Input: part model. Units: mm. Frame: model coordinates. A direction names the side the tool comes from. Round coordinates to 2 decimals unless told otherwise and drop trailing zeros. Order: outer loops, then holes, each group sorted by start corner. A loop starts at its lowest first (then second) coordinate and runs counter-clockwise, first axis right, second up. Notation, with made-up numbers: (59.25, 27) -> (68.25, 27) arc R23 ccw to (68.25, 47) -> close; hole circle Ø9 at (31, 87). An arc over 180 degrees is marked (long way). Use a Markdown table: item, result.
from build123d import *

# Parameters (mm, degrees)
SKETCH1_W           = 42
SKETCH1_H           = 47
BOSS_EXTRUDE1_DEPTH = 5
SKETCH4_W           = 42
SKETCH4_H           = 45
BOSS_EXTRUDE2_DEPTH = 5
BOSS_EXTRUDE3_DEPTH = 3
BOSS_EXTRUDE4_DEPTH = 3
SKETCH2_R           = 2.5
SKETCH2_R_2         = 4.5
CUT_EXTRUDE1_DEPTH  = 54.415821626
SKETCH9_R           = 2
CUT_EXTRUDE4_DEPTH  = 69.373971656
CHAMFER2_SIZE       = 3
CUT_EXTRUDE5_REACH  = 73.903
SKETCH10_R          = 1.5


with BuildPart() as part:
    # Sketch1 → Boss-Extrude1 (new body)
    with BuildSketch(Plane(origin=(0, 0, 0), x_dir=(1, 0, 0), z_dir=(0, 1, 0))):
        Rectangle(SKETCH1_W, SKETCH1_H)
    extrude(amount=BOSS_EXTRUDE1_DEPTH)

    # Sketch4 → Boss-Extrude2 (add)
    with BuildSketch(Plane(origin=(0, 0, -23.5), x_dir=(-1, 0, 0), z_dir=(0, 0, -1))):
        with Locations((0, 22.5)):
            Rectangle(SKETCH4_W, SKETCH4_H)
    extrude(amount=BOSS_EXTRUDE2_DEPTH)

    # Sketch5 → Boss-Extrude3 (add)
    with BuildSketch(Plane(origin=(21, 0, 0), x_dir=(0, 0, -1), z_dir=(1, 0, 0))):
        Polygon((23.5, 13), (15.5, 5), (23.5, 5), align=None)
    extrude(amount=-BOSS_EXTRUDE3_DEPTH)

    # Sketch6 → Boss-Extrude4 (add)
    with BuildSketch(Plane.ZY.offset(21)):
        Polygon((-23.5, 13), (-15.5, 5), (-23.5, 5), align=None)
    extrude(amount=-BOSS_EXTRUDE4_DEPTH)

    # Sketch2 → Cut-Extrude1 (cut, through all)
    with BuildSketch(Plane(origin=(0, 5, 0), x_dir=(1, 0, 0), z_dir=(0, 1, 0))):
        with Locations(Location((-13.081475452, 10.581475452, 0), (0, 0, 270))):
            Circle(SKETCH2_R)
        with Locations(Location((13.081475452, -15.581475452, 0), (0, 0, 270))):
            Circle(SKETCH2_R)
        with Locations(Location((0, -2.5, 0), (0, 0, 270))):
            Circle(SKETCH2_R_2)
    extrude(amount=-CUT_EXTRUDE1_DEPTH, mode=Mode.SUBTRACT)

    # Sketch9 → Cut-Extrude4 (cut, through all)
    with BuildSketch(Plane.XY.offset(-23.5)):
        with Locations((-12.5, 37.5)):
            Circle(SKETCH9_R)
        with Locations((12.5, 37.5)):
            Circle(SKETCH9_R)
        with Locations((12.5, 12.5)):
            Circle(SKETCH9_R)
        with Locations((-12.5, 12.5)):
            Circle(SKETCH9_R)
    extrude(amount=-CUT_EXTRUDE4_DEPTH, mode=Mode.SUBTRACT)

    # Chamfer2
    chamfer2_edges = [part.edges().sort_by_distance(p)[0] for p in [
        (-21, 2.5, 23.5),
        (21, 2.5, 23.5),
        (21, 45, -26),
        (-21, 45, -26),
    ]]
    chamfer(chamfer2_edges, length=CHAMFER2_SIZE)

    # Sketch10 → Cut-Extrude5 (cut, up to next)
    with BuildSketch(Plane(origin=(0, 0, -28.5), x_dir=(-1, 0, 0), z_dir=(0, 0, -1)), mode=Mode.PRIVATE) as cut_extrude5_sk1:
        with Locations((0, 25)):
            Circle(SKETCH10_R)
    cut_extrude5_tool1 = extrude(cut_extrude5_sk1.sketch, amount=-CUT_EXTRUDE5_REACH, mode=Mode.PRIVATE) & part.part
    # Sketch10 → Cut-Extrude5 (cut, up to next)
    with BuildSketch(Plane(origin=(0, 0, -28.5), x_dir=(-1, 0, 0), z_dir=(0, 0, -1)), mode=Mode.PRIVATE) as cut_extrude5_sk2:
        with Locations((0, 10)):
            Circle(SKETCH10_R)
    cut_extrude5_tool2 = extrude(cut_extrude5_sk2.sketch, amount=-CUT_EXTRUDE5_REACH, mode=Mode.PRIVATE) & part.part
    # Sketch10 → Cut-Extrude5 (cut, up to next)
    with BuildSketch(Plane(origin=(0, 0, -28.5), x_dir=(-1, 0, 0), z_dir=(0, 0, -1)), mode=Mode.PRIVATE) as cut_extrude5_sk3:
        with Locations((0, 40)):
            Circle(SKETCH10_R)
    cut_extrude5_tool3 = extrude(cut_extrude5_sk3.sketch, amount=-CUT_EXTRUDE5_REACH, mode=Mode.PRIVATE) & part.part
    add(cut_extrude5_tool1.solids().sort_by_distance((0, 25, -28.5))[0], mode=Mode.SUBTRACT)
    add(cut_extrude5_tool2.solids().sort_by_distance((0, 10, -28.5))[0], mode=Mode.SUBTRACT)
    add(cut_extrude5_tool3.solids().sort_by_distance((0, 40, -28.5))[0], mode=Mode.SUBTRACT)


solid = part.part
1) Cut plane C-C on y = 3.5. Return loops of the section in (x, z), and give its area (3 significant figures).
Answer key:
| item | result |
|---|---|
| outline | (-21, -28.5) -> (21, -28.5) -> (21, 20.5) -> (18, 23.5) -> (-18, 23.5) -> (-21, 20.5) -> close; hole circle Ø5 at (-13.08, -10.58); hole circle Ø9 at (0, 2.5); hole circle Ø5 at (13.08, 15.58) |
| area | 2,070 mm^2 |
2) Draft query along Y for faces 1 (the face through (19, 44, -26)), 2 (the face through (0.325, 38.536, -26.035)), 3 (the face through (-18, 7, -21)), 4 (the face through (12.24, 14.483, -25.965)). Return one class per face: released by +Y, released by -Y, zero draft, split by the parting line, or undercut.
Answer key:
| item | result |
|---|---|
| face 1 | released by +Y |
| face 2 | undercut |
| face 3 | zero draft |
| face 4 | undercut |
3) Set-up query: faces 5 (the face through (-5, 5, 0)), 6 (the face through (-12.934, 35.548, -25.965)). Return all of +Z, -Z, +X, -X, +Y, -Y with unobstructed straight access to the full face (end or side cutting, diameter ignored); none if empty.
Answer key:
| item | result |
|---|---|
| face 5 | +Z, +Y |
| face 6 | +Z, -Z |
4) Cut plane A-A on z = 2.5. Return loops of the section in (x, y), and give its area (3 significant figures).
Answer key:
| item | result |
|---|---|
| outline | (-21, 0) -> (-4.5, 0) -> (-4.5, 5) -> (-21, 5) -> close; (4.5, 0) -> (21, 0) -> (21, 5) -> (4.5, 5) -> close |
| area | 165 mm^2 |
5) Cut plane D-D on z = -7. Return loops of the section in (x, y).
Answer key:
| item | result |
|---|---|
| outline | (-21, 0) -> (21, 0) -> (21, 5) -> (-21, 5) -> close |
6) Ray query, probe 1 along Y at (x, z) = (12.5, -26.25); probe 2 along Y at (x, z) = (0, -26.2); probe 3 along Y at (x, z) = (12, -26). Return the intervals inside material, ascending.
Answer key:
| item | result |
|---|---|
| probe 1 | y = 0 to 10.5, 14.5 to 35.5, 39.5 to 45 |
| probe 2 | y = 0 to 8.5, 11.5 to 23.5, 26.5 to 38.5, 41.5 to 45 |
| probe 3 | y = 0 to 10.56, 14.44 to 35.56, 39.44 to 45 |
7) Cut plane B-B on y = 25. Return loops of the section in (x, z), and give its area (3 significant figures).
Answer key:
| item | result |
|---|---|
| outline | (-21, -28.5) -> (-1.5, -28.5) -> (-1.5, -23.5) -> (-21, -23.5) -> close; (1.5, -28.5) -> (21, -28.5) -> (21, -23.5) -> (1.5, -23.5) -> close |
| area | 195 mm^2 |
8) Contact query for flat-ended pins moving along their axis: P1, Ø5, axis at x = 0, y = 10, coming from the +Z side; P2, Ø12.5, axis at x = 8, z = 7, coming from the +Y side. Output: stop coordinate, or through.
Answer key:
| item | result |
|---|---|
| P1 | stops at z = -23.5 |
| P2 | stops at y = 5 |
